```python
from build123d import *

# Parameters (mm, degrees)
BOSS_EXTRUDE1_DEPTH = 21.4
SKETCH3_R           = 5
CUT_EXTRUDE1_DEPTH  = 24.9
SKETCH4_R           = 1.99
CUT_EXTRUDE2_DEPTH  = 2
SKETCH5_R           = 0.8
CUT_EXTRUDE3_DEPTH  = 26.16346558


with BuildPart() as part:
    # Sketch2 → Boss-Extrude1 (new body)
    with BuildSketch(Plane(origin=(0, 0, 0), x_dir=(1, 0, 0), z_dir=(0, 1, 0))):
        with BuildLine():
            Line((0, 7.8), (-2, 7.8))
            Line((-2, 7.8), (-2, 5.656854249))
            ThreePointArc((-2, 5.656854249), (0, -6), (2, 5.656854249))
            Line((2, 5.656854249), (2, 7.8))
            Line((2, 7.8), (0, 7.8))
        make_face()
    extrude(amount=BOSS_EXTRUDE1_DEPTH)

    # Sketch3 → Cut-Extrude1 (cut)
    with BuildSketch(Plane(origin=(0, 21.4, 0), x_dir=(1, 0, 0), z_dir=(0, 1, 0))):
        with Locations(Location((0, 0, 0), (0, 0, 270))):
            Circle(SKETCH3_R)
    extrude(amount=-CUT_EXTRUDE1_DEPTH, mode=Mode.SUBTRACT)

    # Sketch4 → Cut-Extrude2 (cut)
    with BuildSketch(Plane(origin=(0, 0, -7.8), x_dir=(-1, 0, 0), z_dir=(0, 0, -1))):
        with Locations((0, 11.554448974)):
            Circle(SKETCH4_R)
    extrude(amount=-CUT_EXTRUDE2_DEPTH, mode=Mode.SUBTRACT)

    # Sketch5 → Cut-Extrude3 (cut, through all)
    with BuildSketch(Plane(origin=(0, 0, -5.8), x_dir=(-1, 0, 0), z_dir=(0, 0, -1))):
        with Locations((0, 11.554448974)):
            Circle(SKETCH5_R)
    extrude(amount=-CUT_EXTRUDE3_DEPTH, mode=Mode.SUBTRACT)


solid = part.part
```
Input: part model. Units: mm. Frame: model coordinates. A direction names the side the tool comes from. Coordinates: 2 decimals unless noted, no trailing zeros. Write each loop counter-clockwise with the first axis right and the second up, starting at its lowest first coordinate (ties: lowest second). Pieces come first, ordered by that corner, then holes. Notation, with made-up numbers: (79, -21.5) - (138, -21.5) arc R21 cw to (138, -13.5) - close; hole circle Ø3 at (-36, -20). An arc over 180 degrees is marked (long way). Put each result on its own line as item: value. Start each with the question number.
1) Cut plane A-A (x = 0). Return the cut outline in (y, z), plus the area to 3 significant figures.
2) Reachability of faces 4 (the face through (-2, 0, -5)), 5 (the face through (2, 10.6, -6.7)), 6 (the face through (-1, 12, -5.8)), 7 (the face through (-2, 10.6, -6.7)) from +Z, -Z, +X, -X, +Y, -Y: full face, straight path, thin tool, end or side. Return the list, or none.
3) Cut plane B-B (z = 0). Return the cut outline in (x, y), plus the area to 3 significant figures.
4) Cut plane D-D (x = 3). Return the cut outline in (y, z).
5) Contact query for flat-ended pins moving along their axis: pin 1 (1.1 mm diameter, centred on y = 10, z = -6.5, fed in from -X); pin 2 (1.5 mm diameter, centred on x = 2.5, y = 16.5, fed in from +Z); pin 3 (1.8 mm diameter, centred on x = 0, y = 11.55, fed in from +Z); pin 4 (5 mm diameter, centred on y = 13, z = 3, fed in from +X). Output: stop coordinate, or through.
6) Ray query, L1, parallel to Y at x = 0, z = -5.05; L2, parallel to X at y = 16.25, z = -0.25; L3, parallel to Z at x = 0, y = 13.75. Return the intervals inside material, ascending.
7) Mould query, pull axis Y, two halves, no side actions, for faces 1 (the face through (-0.235, 10.55, 5.995)), 2 (the face through (-1.07, 13.23, -6.81)), 3 (the face through (-2, 21.4, -5)). Classes: pulls with the +Y half, pulls with the -Y half, needs draft (parallel to the pull), parting line crosses it, or undercut.
8) Cut plane C-C (y = 7). Return the cut outline in (x, z), plus the area to 3 significant figures.
Resolved:
1. outline: (0, -7.8) - (9.56, -7.8) - (9.56, -5.8) - (10.75, -5.8) - (10.75, -5) - (0, -5) - close; (0, 5) - (10.75, 5) - (10.75, 6) - (0, 6) - close; (12.35, -5.8) - (13.54, -5.8) - (13.54, -7.8) - (21.4, -7.8) - (21.4, -5) - (12.35, -5) - close; (12.35, 5) - (21.4, 5) - (21.4, 6) - (12.35, 6) - close
1. area: 70.5 mm2
2. face 4: +Z, -Z, +X, -X, -Y
2. face 5: -Z, +X, +Y, -Y
2. face 6: -Z
2. face 7: -Z, -X, +Y, -Y
3. outline: (-6, 0) - (-5, 0) - (-5, 21.4) - (-6, 21.4) - close; (5, 0) - (6, 0) - (6, 21.4) - (5, 21.4) - close
3. area: 42.8 mm2
4. outline: (0, -5.2) - (21.4, -5.2) - (21.4, -4) - (0, -4) - close; (0, 4) - (21.4, 4) - (21.4, 5.2) - (0, 5.2) - close
5. pin 1: stops at x = -2
5. pin 2: stops at z = 5.74
5. pin 3: stops at z = 6
5. pin 4: stops at x = 5.98
6. L1: y = 0 to 10.75, 12.35 to 21.4
6. L2: x = -5.99 to -4.99, 4.99 to 5.99
6. L3: z = -7.8 to -5, 5 to 6
7. face 1: needs draft
7. face 2: undercut
7. face 3: pulls with the +Y half
8. outline: (-2, -7.8) - (2, -7.8) - (2, -5.66) arc R6 ccw (long way) to (-2, -5.66) - close; hole circle Ø10 at (0, 0)
8. area: 42.2 mm2
